```python
from build123d import *

# Parameters (mm, degrees)
BOSS_EXTRU_1_REACH      = 49.343
ESQUISSE4_R             = 1
BOSS_EXTRU_2_REACH      = 47.137
ESQUISSE5_R             = 3.15
ESQUISSE6_R             = 5.15
ENL_V_MAT_EXTRU_2_DEPTH = 22
ESQUISSE8_R             = 3.15
ENL_V_MAT_EXTRU_3_DEPTH = 46.13729057
ESQUISSE9_R             = 5.5
ENL_V_MAT_EXTRU_5_DEPTH = 22
ESQUISSE10_R            = 4.25
ESQUISSE10_R_2          = 3
BOSS_EXTRU_3_DEPTH      = 8
ESQUISSE11_R            = 1.5
ENL_V_MAT_EXTRU_6_DEPTH = 53.396326275
ESQUISSE12_R            = 1
ENL_V_MAT_EXTRU_7_DEPTH = 53.396326275
ENL_V_START             = -3.3
ESQUISSE13_R            = 3
ESQUISSE13_R_2          = 2.1
ENL_V_MAT_EXTRU_8_DEPTH = 3.3


with BuildPart() as part:
    # Esquisse1 → Révolution1 (revolve)
    with BuildSketch(Plane.XY, mode=Mode.PRIVATE) as r_volution1_sk:
        with BuildLine():
            Line((0, 0), (16, 0))
            ThreePointArc((16, 0), (17.693443908, 11.801567412), (23.25, 22.35))
            Line((23.25, 22.35), (27.25, 22.35))
            Line((27.25, 22.35), (27.25, 27.5))
            Line((27.25, 27.5), (26.25, 27.5))
            Line((26.25, 27.5), (26.25, 23.5))
            Line((26.25, 23.5), (22.243806548, 23.5))
            ThreePointArc((22.243806548, 23.5), (16.561622355, 13.136173942), (14.489048167, 1.5))
            Line((14.489048167, 1.5), (0, 1.5))
            Line((0, 1.5), (0, 0))
        make_face()
    revolve(r_volution1_sk.sketch.rotate(Axis((0, 0, 0), (0, 1, 0)), 90), axis=Axis((0, 0, 0), (0, 1, 0)))

    # Esquisse4 → Boss.-Extru.1 (add, up to next)
    with BuildSketch(Plane(origin=(0, 27.5, 0), x_dir=(1, 0, 0), z_dir=(0, 1, 0)), mode=Mode.PRIVATE) as boss_extru_1_sk1:
        with BuildLine():
            Line((-3.575, 26.005420108), (-3.575, 23.5))
            ThreePointArc((-3.575, 23.5), (0, 19.925), (3.575, 23.5))
            Line((3.575, 23.5), (3.575, 26.005420108))
            ThreePointArc((3.575, 26.005420108), (0, 26.25), (-3.575, 26.005420108))
        make_face()
        with Locations(Location((0, 23.5, 0), (0, 0, 270))):
            Circle(ESQUISSE4_R, mode=Mode.SUBTRACT)
    boss_extru_1_tool1 = extrude(boss_extru_1_sk1.sketch, amount=-BOSS_EXTRU_1_REACH, mode=Mode.PRIVATE) - part.part
    # Esquisse4 → Boss.-Extru.1 (add, up to next)
    with BuildSketch(Plane(origin=(0, 27.5, 0), x_dir=(1, 0, 0), z_dir=(0, 1, 0)), mode=Mode.PRIVATE) as boss_extru_1_sk2:
        with BuildLine():
            Line((-3.575, -23.5), (-3.575, -26.005420108))
            ThreePointArc((-3.575, -26.005420108), (0, -26.25), (3.575, -26.005420108))
            Line((3.575, -26.005420108), (3.575, -23.5))
            ThreePointArc((3.575, -23.5), (0, -19.925), (-3.575, -23.5))
        make_face()
        with Locations(Location((0, -23.5, 0), (0, 0, 270))):
            Circle(ESQUISSE4_R, mode=Mode.SUBTRACT)
    boss_extru_1_tool2 = extrude(boss_extru_1_sk2.sketch, amount=-BOSS_EXTRU_1_REACH, mode=Mode.PRIVATE) - part.part
    add(boss_extru_1_tool1.solids().sort_by_distance((0, 27.5, -26.154539))[0])
    add(boss_extru_1_tool2.solids().sort_by_distance((3.479539, 27.5, 24.75271))[0])

    # Esquisse5 → Boss.-Extru.2 (add, up to next)
    with BuildSketch(Plane(origin=(0, 23.5, 0), x_dir=(1, 0, 0), z_dir=(0, 1, 0)), mode=Mode.PRIVATE) as boss_extru_2_sk1:
        with BuildLine():
            Line((-16.55, 7.5), (-20.941273355, 7.5))
            ThreePointArc((-20.941273355, 7.5), (-22.243806548, 0), (-20.941273355, -7.5))
            Line((-20.941273355, -7.5), (-16.55, -7.5))
            ThreePointArc((-16.55, -7.5), (-9.05, 0), (-16.55, 7.5))
        make_face()
        with Locations(Location((-16.55, 0, 0), (0, 0, 270))):
            Circle(ESQUISSE5_R, mode=Mode.SUBTRACT)
    boss_extru_2_tool1 = extrude(boss_extru_2_sk1.sketch, amount=-BOSS_EXTRU_2_REACH, mode=Mode.PRIVATE) - part.part
    # Esquisse5 → Boss.-Extru.2 (add, up to next)
    with BuildSketch(Plane(origin=(0, 23.5, 0), x_dir=(1, 0, 0), z_dir=(0, 1, 0)), mode=Mode.PRIVATE) as boss_extru_2_sk2:
        with BuildLine():
            Line((16.55, -7.5), (20.941273355, -7.5))
            ThreePointArc((20.941273355, -7.5), (22.243806548, 0), (20.941273355, 7.5))
            Line((20.941273355, 7.5), (16.55, 7.5))
            ThreePointArc((16.55, 7.5), (9.05, 0), (16.55, -7.5))
        make_face()
        with Locations(Location((16.55, 0, 0), (0, 0, 224.870853296))):
            Circle(ESQUISSE5_R, mode=Mode.SUBTRACT)
    boss_extru_2_tool2 = extrude(boss_extru_2_sk2.sketch, amount=-BOSS_EXTRU_2_REACH, mode=Mode.PRIVATE) - part.part
    add(boss_extru_2_tool1.solids().sort_by_distance((-18.745637, 23.5, -7.300231))[0])
    add(boss_extru_2_tool2.solids().sort_by_distance((18.745637, 23.5, 7.300231))[0])

    # Esquisse6 → Enlèv. mat.-Extru.2 (cut)
    with BuildSketch(Plane.XZ):
        with Locations(Location((0, 0, 0), (0, 0, 270))):
            Circle(ESQUISSE6_R)
    extrude(amount=-ENL_V_MAT_EXTRU_2_DEPTH, mode=Mode.SUBTRACT)

    # Esquisse8 → Enlèv. mat.-Extru.3 (cut, through all)
    with BuildSketch(Plane(origin=(0, 23.5, 0), x_dir=(1, 0, 0), z_dir=(0, 1, 0))):
        with Locations(Location((-16.55, 0, 0), (0, 0, 270))):
            Circle(ESQUISSE8_R)
        with Locations(Location((16.55, 0, 0), (0, 0, 254.52201619))):
            Circle(ESQUISSE8_R)
    extrude(amount=-ENL_V_MAT_EXTRU_3_DEPTH, mode=Mode.SUBTRACT)

    # Esquisse9 → Enlèv. mat.-Extru.5 (cut)
    with BuildSketch(Plane(origin=(0, 0, 0), x_dir=(-1, 0, 0), z_dir=(0, -1, 0))):
        with Locations(Location((16.55, 0, 0), (0, 0, 90))):
            Circle(ESQUISSE9_R)
        with Locations(Location((-16.55, 0, 0), (0, 0, 74.662665416))):
            Circle(ESQUISSE9_R)
    extrude(amount=-ENL_V_MAT_EXTRU_5_DEPTH, mode=Mode.SUBTRACT)

    # Esquisse10 → Boss.-Extru.3 (add)
    with BuildSketch(Plane.XZ):
        with Locations(Location((-8.396893027, 8.396893027, 0), (0, 0, 118.784200872))):
            Circle(ESQUISSE10_R)
        with Locations(Location((8.40042856, 8.40042856, 0), (0, 0, 270))):
            Circle(ESQUISSE10_R_2)
        with Locations(Location((8.40042856, -8.40042856, 0), (0, 0, 90))):
            Circle(ESQUISSE10_R)
        with Locations(Location((-8.396893027, -8.396893027, 0), (0, 0, 270))):
            Circle(ESQUISSE10_R_2)
    extrude(amount=BOSS_EXTRU_3_DEPTH)

    # Esquisse11 → Enlèv. mat.-Extru.6 (cut, through all)
    with BuildSketch(Plane.XZ.offset(8)):
        with Locations(Location((-8.396893027, 8.396893027, 0), (0, 0, 270))):
            Circle(ESQUISSE11_R)
        with Locations(Location((8.40042856, -8.40042856, 0), (0, 0, 270))):
            Circle(ESQUISSE11_R)
    extrude(amount=-ENL_V_MAT_EXTRU_6_DEPTH, mode=Mode.SUBTRACT)

    # Esquisse12 → Enlèv. mat.-Extru.7 (cut, through all)
    with BuildSketch(Plane.XZ.offset(8)):
        with Locations(Location((-8.396893027, -8.396893027, 0), (0, 0, 270))):
            Circle(ESQUISSE12_R)
        with Locations(Location((8.40042856, 8.40042856, 0), (0, 0, 270))):
            Circle(ESQUISSE12_R)
    extrude(amount=-ENL_V_MAT_EXTRU_7_DEPTH, mode=Mode.SUBTRACT)

    # Esquisse13 → Enlèv. mat.-Extru.8 (cut)
    # profile 1 of 2: a face of its own
    with BuildSketch(Plane.XZ.offset(8).offset(ENL_V_START)):
        with Locations(Location((-8.396893027, -8.396893027, 0), (0, 0, 270))):
            Circle(ESQUISSE13_R)
        with Locations(Location((-8.396893027, -8.396893027, 0), (0, 0, 270))):
            Circle(ESQUISSE13_R_2, mode=Mode.SUBTRACT)
    # profile 2 of 2: a face of its own
    with BuildSketch(Plane.XZ.offset(8).offset(ENL_V_START)):
        with Locations(Location((8.40042856, 8.40042856, 0), (0, 0, 270))):
            Circle(ESQUISSE13_R)
        with Locations(Location((8.40042856, 8.40042856, 0), (0, 0, 270))):
            Circle(ESQUISSE13_R_2, mode=Mode.SUBTRACT)
    extrude(amount=ENL_V_MAT_EXTRU_8_DEPTH, mode=Mode.SUBTRACT)


solid = part.part
```
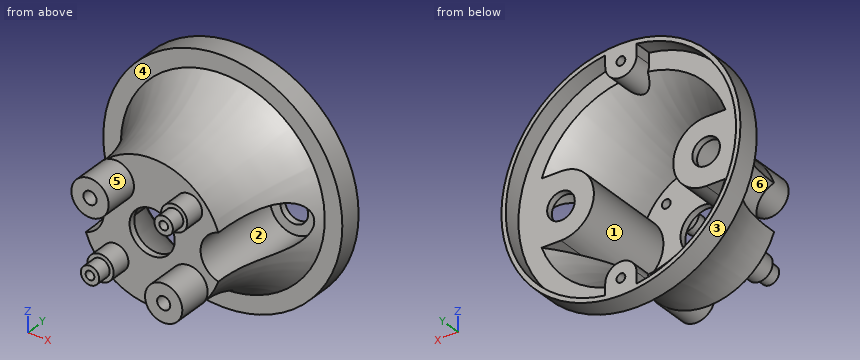
Here's how the part is built. I have some questions about the finished solid (model axes, mm). Face numbers are marked on the shaded views. A direction names the side the tool comes from. Coordinates: 2 decimals unless noted, no trailing zeros. Write each loop counter-clockwise with the first axis right and the second up, starting at its lowest first coordinate (ties: lowest second). Pieces come first, ordered by that corner, then holes. Notation, with made-up numbers: (10.25, 72.25) -> (44.25, 72.25) arc R23 cw to (44.25, 111.25) -> close; hole circle Ø6 at (58, 2). An arc over 180 degrees is marked (long way). Use a Markdown table: item, result. Add a question column.
(1) Please list where these lines run through material, in increasing order: line 1 (X direction, y = 6, z = 0); line 2 (Z direction, x = -13.5, y = 12.5); line 3 (Z direction, x = 5, y = 6).
(2) If we section it at D-D, the plane y = 19: Write out the boundary of the cut face in (x, z).
(3) If we section it at C-C, the plane y = 15: Write out the boundary of the cut face in (x, z).
(4) If we section it at B-B, the plane y = 8: Write out the boundary of the cut face in (x, z).
(5) For the marked faces 1 and 2, which set-ups out of +Z, -Z, +X, -X, +Y, -Y let a thin tool reach every point of the face, with its end or its side?
(6) We'd pull the mould along X, two halves only. Please class the marked faces 3, 4, 5 and 6: +X half, -X half, draft (parallel to the pull), parting line (faces both ways), or undercut.
(7) If we section it at A-A, the plane x = 0: Write out the boundary of the cut face in (y, z) (3 decimals), and give its area (3 significant figures).
(8) I'm going to push flat-ended pins straight in: P1, Ø8, axis at x = -3, z = -7, coming from the +Y side; P2, Ø3, axis at x = 6.5, y = 18.5, coming from the +Z side; P3, Ø5, axis at x = 16, y = 3, coming from the -Z side. Where does each tip first touch, or does it pass through?
Outcome:
| question | item | result |
|---|---|---|
| 1 | line 1 | x = -11.05 to -9.05, 9.05 to 11.05 |
| 1 | line 2 | z = -11.8 to -9.21, -6.85 to -4.58, 4.58 to 6.85, 9.21 to 11.8 |
| 1 | line 3 | z = -15.56 to -13.96, 13.96 to 15.56 |
| 2 | outline | (-20.64, -3.67) arc R20.97 ccw to (20.64, -3.67) arc R5.5 cw (long way) to (20.64, 3.67) arc R20.97 ccw to (-20.64, 3.67) arc R5.5 cw (long way) to start; hole (-17.71, -7.5) arc R19.23 ccw to (17.71, -7.5) -> (16.55, -7.5) arc R7.5 cw to (16.55, 7.5) -> (17.71, 7.5) arc R19.23 ccw to (-17.71, 7.5) -> (-16.55, 7.5) arc R7.5 cw to (-16.55, -7.5) -> close |
| 3 | outline | (-18.16, -5.26) arc R18.91 ccw to (18.16, -5.26) arc R5.5 cw (long way) to (18.16, 5.26) arc R18.91 ccw to (-18.16, 5.26) arc R5.5 cw (long way) to start; hole (-15.59, -7.44) arc R17.28 ccw to (15.59, -7.44) arc R7.5 cw to (15.59, 7.44) arc R17.28 ccw to (-15.59, 7.44) arc R7.5 cw to start |
| 4 | outline | (-15.78, -5.45) arc R16.69 ccw to (15.78, -5.45) arc R5.5 cw to (15.78, 5.45) arc R16.69 ccw to (-15.78, 5.45) arc R5.5 cw to start; hole (-13.52, -6.86) arc R15.16 ccw to (13.52, -6.86) arc R7.5 cw to (13.52, 6.86) arc R15.16 ccw to (-13.52, 6.86) arc R7.5 cw to start |
| 5 | face 1 | +Y |
| 5 | face 2 | -Y |
| 6 | face 3 | parting line |
| 6 | face 4 | draft |
| 6 | face 5 | undercut |
| 6 | face 6 | undercut |
| 7 | outline | (0, -16) arc R35 cw to (22.35, -23.25) -> (22.35, -27.25) -> (27.5, -27.25) -> (27.5, -24.5) -> (23.5, -24.5) -> (23.5, -22.5) -> (27.5, -22.5) -> (27.5, -19.925) -> (20.172, -19.925) arc R36.5 ccw to (1.5, -14.489) -> (1.5, -5.15) -> (0, -5.15) -> close; (0, 5.15) -> (1.5, 5.15) -> (1.5, 14.489) arc R36.5 ccw to (20.172, 19.925) -> (27.5, 19.925) -> (27.5, 22.5) -> (23.5, 22.5) -> (23.5, 24.5) -> (27.5, 24.5) -> (27.5, 27.25) -> (22.35, 27.25) -> (22.35, 23.25) arc R35 cw to (0, 16) -> close |
| 7 | area | 162 mm^2 |
| 8 | P1 | stops at y = 1.5 |
| 8 | P2 | stops at z = 20.68 |
| 8 | P3 | stops at z = -8.68 |
